Read the model definition and answer for the solid it produces. Units are mm, in the model's axes. Coordinates: 2 decimals unless noted, no trailing zeros. Loops run counter-clockwise (first coordinate to the right, second up) from the corner with the lowest first, then second, coordinate; pieces in that order, holes last.
from build123d import *

# Parameters (mm, degrees)
EXTRUDE_1_DEPTH     = 6
SKETCH_2_R          = 1.65
CUT_EXTRUDE_1_DEPTH = 6
FILLET_1_R          = 1
CHAMFER_1_SIZE      = 0.5
FILLET_2_R          = 0.5


with BuildPart() as part:
    # 草圖1 → 填料-伸長1 (new body)
    with BuildSketch(Plane(origin=(0, 0, 0), x_dir=(0, 0, -1), z_dir=(1, 0, 0))):
        with BuildLine():
            Line((0, 0), (6.95, 0))
            ThreePointArc((6.95, 0), (8.5, 1.55), (10.05, 0))
            Line((10.05, 0), (12, 0))
            Line((12, 0), (12, 4))
            Line((12, 4), (0, 4))
            Line((0, 4), (0, 0))
        make_face()
    extrude(amount=EXTRUDE_1_DEPTH)

    # 草圖2 → 除料-伸長1 (cut)
    with BuildSketch(Plane(origin=(0, 0, 0), x_dir=(-1, 0, 0), z_dir=(0, -1, 0))):
        with Locations(Location((-3, 3, 0), (0, 0, 90))):
            Circle(SKETCH_2_R)
    extrude(amount=-CUT_EXTRUDE_1_DEPTH, mode=Mode.SUBTRACT)

    # 圓角1
    fillet_1_edges = [part.edges().sort_by_distance(p)[0] for p in [
        (6, 2, -12),
        (6, 2, 0),
        (0, 2, -12),
        (0, 2, 0),
    ]]
    fillet(fillet_1_edges, radius=FILLET_1_R)

    # 導角1
    chamfer_1_edges = [part.edges().sort_by_distance(p)[0] for p in [
        (3, 4, -1.35),
    ]]
    chamfer(chamfer_1_edges, length=CHAMFER_1_SIZE)

    # 圓角2
    fillet_2_edges = [part.edges().sort_by_distance(p)[0] for p in [
        (6, 4, -6),
        (0, 4, -6),
        (3, 4, 0),
        (3, 4, -12),
        (0.292893219, 4, -0.292893219),
        (5.707106781, 4, -0.292893219),
        (0.292893219, 4, -11.707106781),
        (5.707106781, 4, -11.707106781),
    ]]
    fillet(fillet_2_edges, radius=FILLET_2_R)


solid = part.part
Q1. Straight lines are drawn through the part: probe 1 along X at (y, z) = (2.2, -3); probe 2 along Y at (x, z) = (2.85, -8.5); probe 3 along Z at (x, y) = (4.2, 2.6). For each, find the intervals that lie inside material, in ascending order.
Findings below:
probe 1: x = 0 to 1.35, 4.65 to 6
probe 2: y = 1.55 to 4
probe 3: z = -12 to -4.13, -1.87 to 0
Q2. A cutting plane is placed at B-B (z = -3). Give the vertices of the cut face in (x, y), then the cut area to 3 significant figures.
Findings below:
outline: (0, 0) - (1.35, 0) - (1.35, 3.5) - (0.85, 4) - (0.5, 4) arc R0.5 ccw to (0, 3.5) - close; (4.65, 0) - (6, 0) - (6, 3.5) arc R0.5 ccw to (5.5, 4) - (5.15, 4) - (4.65, 3.5) - close
area: 10.4 mm2
Q3. A cutting plane is placed at C-C (x = 3). Give the vertices of the cut face in (y, z), then the cut area to 3 significant figures.
Findings below:
outline: (0, -12) - (3.5, -12) arc R0.5 ccw to (4, -11.5) - (4, -5.15) - (3.5, -4.65) - (0, -4.65) - (0, -6.95) arc R1.55 cw to (0, -10.05) - close; (0, -1.35) - (3.5, -1.35) - (4, -0.85) - (4, -0.5) arc R0.5 ccw to (3.5, 0) - (0, 0) - close
area: 30.7 mm2
Q4. Determine the mould class of faces 1 (the face through (0, 2, -6)), 2 (the face through (2.96, 1.55, -8.47)), 3 (the face through (3, 2, -12)) for opening direction Z: +Z half, -Z half, draft (parallel to the pull), parting line (faces both ways), or undercut.
Findings below:
face 1: draft
face 2: undercut
face 3: -Z half
Q5. A cutting plane is placed at D-D (y = 1.8). Give the vertices of the cut face in (x, z), then the cut area to 3 significant figures.
Findings below:
outline: (0, -11) arc R1 ccw to (1, -12) - (5, -12) arc R1 ccw to (6, -11) - (6, -1) arc R1 ccw to (5, 0) - (1, 0) arc R1 ccw to (0, -1) - close; hole circle Ø3.3 at (3, -3)
area: 62.6 mm2
Q6. A cutting plane is placed at A-A (y = 0.6). Give the vertices of the cut face in (x, z).
Findings below:
outline: (0, -11) arc R1 ccw to (1, -12) - (5, -12) arc R1 ccw to (6, -11) - (6, -9.93) - (0, -9.93) - close; (0, -7.07) - (6, -7.07) - (6, -1) arc R1 ccw to (5, 0) - (1, 0) arc R1 ccw to (0, -1) - close; hole circle Ø3.3 at (3, -3)
